Source: CAD feature listing. Evaluate the final solid. Frame: model axes, mm. A direction names the side the tool comes from. Coordinates: 2 decimals unless noted, no trailing zeros.
Item 1: Ray query, line 1 (Y direction, x = 8, z = 6.75); line 2 (X direction, y = 4.25, z = 0); line 3 (X direction, y = 9.3, z = 0). Return the intervals inside material, ascending.
Item 2: Reachability of faces 1 (the cylindrical face through (-4.289, 4.958, 4.196)), 2 (the flat face through (0, 7.5, 0)), 3 (the flat face through (0, 4.8, 0)), 4 (the flat face through (-0.5, 8, 6.6)) from +Z, -Z, +X, -X, +Y, -Y: full face, straight path, thin tool, end or side. Return the list, or none.
Item 3: Mould query, pull axis X, two halves, no side actions, for faces 5 (the cylindrical face through (2, 5, -8)), 6 (the cylindrical face through (-0.728, 8.768, 1.755)), 7 (the cylindrical face through (6.99, 4.96, 7.15)). Classes: released by +X, released by -X, zero draft, split by the parting line, or undercut.
Item 4: Contact query for flat-ended pins moving along their axis: P1, Ø2, axis at y = 2, z = 3, coming from the -X side; P2, Ø1.2, axis at y = 3.5, z = 7.5, coming from the -X side; P3, Ø2, axis at y = 0.5, z = 9, coming from the -X side. Output: stop coordinate, or through.
from build123d import *

# Parameters (mm, degrees)
SKETCH1_R           = 6
BOSS_EXTRUDE1_DEPTH = 10
SKETCH2_R           = 1.9
CUT_EXTRUDE1_DEPTH  = 2.5
SKETCH3_R           = 3.75
CUT_EXTRUDE2_DEPTH  = 4.8
BOSS_EXTRUDE2_DEPTH = 10
BOSS_EXTRUDE3_DEPTH = 2
BOSS_EXTRUDE5_START = -2
SKETCH9_R           = 1.9
BOSS_EXTRUDE5_DEPTH = 2
CHAMFER1_SIZE       = 1


with BuildPart() as part:
    # Sketch1 → Boss-Extrude1 (new body)
    with BuildSketch(Plane(origin=(0, 0, 0), x_dir=(1, 0, 0), z_dir=(0, 1, 0))):
        with Locations(Location((0, 0, 0), (0, 0, 270))):
            Circle(SKETCH1_R)
    extrude(amount=BOSS_EXTRUDE1_DEPTH)

    # Sketch2 → Cut-Extrude1 (cut)
    with BuildSketch(Plane(origin=(0, 10, 0), x_dir=(1, 0, 0), z_dir=(0, 1, 0))):
        with Locations(Location((0, 0, 0), (0, 0, 270))):
            Circle(SKETCH2_R)
    extrude(amount=-CUT_EXTRUDE1_DEPTH, mode=Mode.SUBTRACT)

    # Sketch3 → Cut-Extrude2 (cut)
    with BuildSketch(Plane.XZ):
        with Locations(Location((0, 0, 0), (0, 0, 270))):
            Circle(SKETCH3_R)
    extrude(amount=-CUT_EXTRUDE2_DEPTH, mode=Mode.SUBTRACT)

    # Sketch5 → Boss-Extrude2 (add)
    with BuildSketch(Plane.XZ):
        with BuildLine():
            Line((0, 6), (0, 10))
            ThreePointArc((0, 10), (7.071067812, 7.071067812), (10, 0))
            ThreePointArc((10, 0), (2, -8), (-6, 0))
            ThreePointArc((-6, 0), (4.242640687, -4.242640687), (0, 6))
        make_face()
    extrude(amount=-BOSS_EXTRUDE2_DEPTH)

    # Sketch7 → Boss-Extrude3 (add)
    with BuildSketch(Plane.XZ):
        with BuildLine():
            Line((-1.5, 11.401754251), (-1.5, 7.348469228))
            ThreePointArc((-1.5, 7.348469228), (-5.809475019, 4.74341649), (-7.5, 0))
            ThreePointArc((-7.5, 0), (2, -9.5), (11.5, 0))
            ThreePointArc((11.5, 0), (7.582875444, 8.645808233), (-1.5, 11.401754251))
        make_face()
        with BuildLine():
            Line((0, 10), (0, 6))
            ThreePointArc((0, 6), (-4.242640687, 4.242640687), (-6, 0))
            ThreePointArc((-6, 0), (2, -8), (10, 0))
            ThreePointArc((10, 0), (7.071067812, 7.071067812), (0, 10))
        make_face(mode=Mode.SUBTRACT)
    extrude(amount=-BOSS_EXTRUDE3_DEPTH)

    # Sketch9 → Boss-Extrude5 (add)
    with BuildSketch(Plane(origin=(0, 10, 0), x_dir=(1, 0, 0), z_dir=(0, 1, 0)).offset(BOSS_EXTRUDE5_START)):
        with BuildLine():
            Line((-1.5, -11.401754251), (-1.5, -7.348469228))
            ThreePointArc((-1.5, -7.348469228), (-5.809475019, -4.74341649), (-7.5, 0))
            ThreePointArc((-7.5, 0), (2, 9.5), (11.5, 0))
            ThreePointArc((11.5, 0), (7.582875444, -8.645808233), (-1.5, -11.401754251))
        make_face()
        with Locations(Location((0, 0, 0), (0, 0, 270))):
            Circle(SKETCH9_R, mode=Mode.SUBTRACT)
    extrude(amount=BOSS_EXTRUDE5_DEPTH)

    # Chamfer1
    chamfer1_edges = [part.edges().sort_by_distance(p)[0] for p in [
        (7.582875444, 2, 8.645808233),
        (2, 2, -9.5),
        (-5.809475019, 2, 4.74341649),
        (-5.809475019, 8, 4.74341649),
        (2, 8, -9.5),
        (7.582875444, 8, 8.645808233),
    ]]
    chamfer(chamfer1_edges, length=CHAMFER1_SIZE)


solid = part.part
Answer list:
1. line 1: y = 0 to 2, 8 to 10
1. line 2: x = -6 to -3.75, 3.75 to 10
1. line 3: x = -7.5 to -1.9, 1.9 to 11.5
2. face 1: +Z, -X
2. face 2: +Y
2. face 3: -Y
2. face 4: none
3. face 5: split by the parting line
3. face 6: undercut
3. face 7: released by +X
4. P1: stops at x = -6.95
4. P2: stops at x = 0
4. P3: stops at x = -1.5
